CAD build for the part. Positions are in the model's coordinates, mm. A direction names the side the tool comes from. Give positions to 0.01 mm unless a question says otherwise; leave off trailing zeros. Loops run counter-clockwise (first coordinate to the right, second up) from the corner with the lowest first, then second, coordinate; pieces in that order, holes last. Notation, with made-up numbers: (7, 39.25) -> (30, 39.25) arc R20 cw to (30, 49.25) -> close; hole circle Ø9 at (44, 1.5). An arc over 180 degrees is marked (long way). Write each question's results on one line, items separated by ' | '. Start each with the question number.
```python
from build123d import *

# Parameters (mm, degrees)
SKETCH_R  = 1.55
PAD_DEPTH = 1


with BuildPart() as part:
    # Sketch → Pad (new body, symmetric)
    with BuildSketch(Plane.XY):
        Polygon((21.5, -10), (21.5, 12), (-21.5, 12), (-21.5, -10), (-15.75, -10), (-15.75, -6.5), (-12.25, -6.5), (-12.25, -10), (-1.9, -10), (-1.9, 7), (1.9, 7), (1.9, -10), (12.25, -10), (12.25, -6.5), (15.75, -6.5), (15.75, -10), align=None)
        with Locations((15, 0)):
            Circle(SKETCH_R, mode=Mode.SUBTRACT)
        with Locations((-15, 0)):
            Circle(SKETCH_R, mode=Mode.SUBTRACT)
    extrude(amount=PAD_DEPTH, both=True)


solid = part.part
```
Q1. Saw through at C-C, the plane z = 0.5. List the corners of the cut face in (x, y), then the cut area to 3 significant figures.
Q2. Saw through at B-B, the plane x = -15. List the corners of the cut face in (y, z), then the cut area to 3 significant figures.
Q3. Wall check: L1, parallel to X at y = -8.5, z = -0.15; L2, parallel to X at y = -2, z = -0.3; L3, parallel to Y at x = 15, z = 0. Give the ranges that are in metal, low to high.
Q4. Which spindle directions (+Z, -Z, +X, -X, +Y, -Y) get a long thin tool onto all of the face, cutting with end or side? Do faces 1 (the face through (7, -10, 0)), 2 (the face through (12.25, -8, 0)). Say none if no direction does.
Q5. Mould opens along Y. For faces 3 (the face through (15.75, -8, 0)), 4 (the face through (-16.55, 0.07, -0.01)), 5 (the face through (13.45, 0.07, -0.01)), 6 (the face through (0, 7, 0)) say: pulls with the +Y half, pulls with the -Y half, needs draft (parallel to the pull), parting line crosses it, or undercut.
Q6. Saw through at D-D, the plane x = -0.5. List the corners of the cut face in (y, z), then the cut area to 3 significant figures.
Q7. Drop a flat-ended pin along its axis: pin 1 (0.6 mm diameter, centred on x = 13, z = -0.5, fed in from -Y). Give the stop position or say it passes through.
Q8. Saw through at A-A, the plane y = 0. List the corners of the cut face in (x, z), then the cut area to 3 significant figures.
Answer block:
1) outline: (-21.5, -10) -> (-15.75, -10) -> (-15.75, -6.5) -> (-12.25, -6.5) -> (-12.25, -10) -> (-1.9, -10) -> (-1.9, 7) -> (1.9, 7) -> (1.9, -10) -> (12.25, -10) -> (12.25, -6.5) -> (15.75, -6.5) -> (15.75, -10) -> (21.5, -10) -> (21.5, 12) -> (-21.5, 12) -> close; hole circle Ø3.1 at (-15, 0); hole circle Ø3.1 at (15, 0) | area: 842 mm2
2) outline: (-6.5, -1) -> (-1.55, -1) -> (-1.55, 1) -> (-6.5, 1) -> close; (1.55, -1) -> (12, -1) -> (12, 1) -> (1.55, 1) -> close | area: 30.8 mm2
3) L1: x = -21.5 to -15.75, -12.25 to -1.9, 1.9 to 12.25, 15.75 to 21.5 | L2: x = -21.5 to -1.9, 1.9 to 21.5 | L3: y = -6.5 to -1.55, 1.55 to 12
4) face 1: +Z, -Z, +X, -X, -Y | face 2: +Z, -Z, -Y
5) face 3: needs draft | face 4: undercut | face 5: undercut | face 6: pulls with the -Y half
6) outline: (7, -1) -> (12, -1) -> (12, 1) -> (7, 1) -> close | area: 10.0 mm2
7) pin 1: stops at y = -6.5
8) outline: (-21.5, -1) -> (-16.55, -1) -> (-16.55, 1) -> (-21.5, 1) -> close; (-13.45, -1) -> (-1.9, -1) -> (-1.9, 1) -> (-13.45, 1) -> close; (1.9, -1) -> (13.45, -1) -> (13.45, 1) -> (1.9, 1) -> close; (16.55, -1) -> (21.5, -1) -> (21.5, 1) -> (16.55, 1) -> close | area: 66.0 mm2
